Can you work these out from the model? Positions are in its coordinate system, mm. A direction names the side the tool comes from. Coordinates: 2 decimals unless noted, no trailing zeros. Order: outer loops, then holes, each group sorted by start corner. A loop starts at its lowest first (then second) coordinate and runs counter-clockwise, first axis right, second up. Notation, with made-up numbers: (64.25, 30.5) -> (90.25, 30.5) arc R33 ccw to (90.25, 62.5) -> close; hole circle Ø10 at (32.25, 33.5). An arc over 180 degrees is marked (long way). Write item = value, one per line. Start each with the question number.
Autodesk Inventor part; units mm, degrees
ref_plane "YZ Plane" through (0, 0, 0) normal (1, 0, 0) x (0, 1, 0)
ref_plane "XZ Plane" through (0, 0, 0) normal (0, 1, 0) x (-1, 0, 0)
ref_plane "XY Plane" through (0, 0, 0) normal (0, 0, 1) x (1, 0, 0)
sketch "Sketch1" plane through (0, 0, 0) normal (0, 1, 0) x (-1, 0, 0)
  circle A0 centre (25.2, -7) radius 1.35
  circle A1 centre (17.7, -7) radius 0.65
  circle A2 centre (15.2, -7) radius 0.65
  circle A3 centre (12.7, -7) radius 0.65
  line L0 (10, -7) -> (10, -8)
  line L1 (13, -11) -> (26, -11)
  line L2 (26, -3) -> (13, -3)
  line L3 (10, -6) -> (10, -7)
  arc A4 (13, -3) -> (10, -6) centre (13, -6) ccw
  arc A5 (10, -8) -> (13, -11) centre (13, -8) ccw
  line L4 (29, -14) -> (29, -18)
  line L5 (31, -20) -> (78, -20)
  line L6 (80, -18) -> (80, 4)
  line L7 (78, 6) -> (31, 6)
  line L8 (29, 4) -> (29, 0)
  arc A6 (26, -3) -> (29, 0) centre (26, 0) ccw
  arc A7 (29, -14) -> (26, -11) centre (26, -14) ccw
  arc A8 (31, 6) -> (29, 4) centre (31, 4) ccw
  arc A9 (80, 4) -> (78, 6) centre (78, 4) ccw
  arc A10 (78, -20) -> (80, -18) centre (78, -18) ccw
  arc A11 (29, -18) -> (31, -20) centre (31, -18) ccw
  point P0 (0, 0)
  point P1 (10, -3)
  point P2 (29, -7)
  point P3 (29, -20)
  point P4 (80, -20)
  point P5 (80, 6)
  point P6 (29, 6)
  dimension "d0" = 2.7
  dimension "d1" = 1.3
  dimension "d2" = 1.3
  dimension "d3" = 1.3
  dimension "d4" = 3
  dimension "d5" = 13
  dimension "d6" = 51
  dimension "d7" = 26
  dimension "d8" = 3
  dimension "d9" = 2
extrude "Extrusion1" add sketch "Sketch1" along normal blind 3
sketch "Sketch2" plane through (0, 3, 0) normal (0, 1, 0) x (1, 0, 0)
  line L0 (-77, 17) -> (-32, 17)
  line L1 (-32, 17) -> (-32, -3)
  line L2 (-32, -3) -> (-77, -3)
  line L3 (-77, -3) -> (-77, 17)
  line L4 (-78, 20) -> (-31, 20)
  line L5 (-29, 18) -> (-29, -4)
  line L6 (-41, -6) -> (-68, -6)
  line L7 (-80, -4) -> (-80, 18)
  arc A0 (-78, 20) -> (-80, 18) centre (-78, 18) ccw
  arc A1 (-29, 18) -> (-31, 20) centre (-31, 18) ccw
  arc A2 (-31, -6) -> (-29, -4) centre (-31, -4) ccw
  arc A3 (-80, -4) -> (-78, -6) centre (-78, -4) ccw
  line L8 (-77, -3) -> (-75.5, -3)
  line L9 (-75.5, -3) -> (-75.5, -1.5)
  circle A4 centre (-75.5, -1.5) radius 1
  line L10 (-32, 17) -> (-33.5, 17)
  line L11 (-33.5, 17) -> (-33.5, 15.5)
  circle A5 centre (-33.5, 15.5) radius 1
  line L12 (-49.42, 17) -> (-59.58, 17)
  line L13 (-59.58, 17) -> (-59.58, 14.46)
  line L14 (-59.58, 14.46) -> (-49.42, 14.46)
  line L15 (-49.42, 14.46) -> (-49.42, 17)
  line L16 (-78, -6) -> (-31, -6)
  line L17 (-77, -6) -> (-71, -6)
  line L18 (-71, -9) -> (-71, -9)
  line L19 (-74, -12) -> (-74, -12)
  line L20 (-77, -9) -> (-77, -6)
  line L21 (-32, -6) -> (-38, -6)
  line L22 (-38, -9) -> (-38, -9)
  line L23 (-35, -12) -> (-35, -12)
  line L24 (-32, -9) -> (-32, -6)
  arc A6 (-77, -9) -> (-74, -12) centre (-74, -9) ccw
  arc A7 (-74, -12) -> (-71, -9) centre (-74, -9) ccw
  arc A8 (-68, -6) -> (-71, -9) centre (-68, -9) ccw
  arc A9 (-38, -9) -> (-41, -6) centre (-41, -9) ccw
  arc A10 (-38, -9) -> (-35, -12) centre (-35, -9) ccw
  arc A11 (-35, -12) -> (-32, -9) centre (-35, -9) ccw
  circle A12 centre (-74, -9) radius 1.5
  circle A13 centre (-35, -9) radius 1.5
  line L25 (-77, -6) -> (-68, -6)
  line L26 (-41, -6) -> (-32, -6)
  point P0 (0, 0)
  point P1 (-38, -12)
  dimension "d12" = 45
  dimension "d13" = 20
  dimension "d14" = 2
  dimension "d15" = 1.5
  dimension "d16" = 1.5
  dimension "d17" = 2
  dimension "d18" = 1.5
  dimension "d19" = 1.5
  dimension "d20" = 2
  dimension "d22" = 10.16
  dimension "d23" = 2.54
  dimension "d24" = 3
  dimension "d25" = 3
  dimension "d26" = 3
extrude "Extrusion2" add sketch "Sketch2" against normal blind 3 contours L16 A8 A7 A6 L20 | L24 A11 A10 A9 L16
sketch "Sketch3" plane through (0, 3, 0) normal (0, 1, 0) x (1, 0, 0)
  line L0 (-77, 17) -> (-32, 17)
  line L1 (-32, 17) -> (-32, -3)
  line L2 (-32, -3) -> (-77, -3)
  line L3 (-77, -3) -> (-77, 17)
  line L4 (-78, 20) -> (-31, 20)
  line L5 (-29, 18) -> (-29, -4)
  line L6 (-41, -6) -> (-68, -6)
  line L7 (-80, -4) -> (-80, 18)
  arc A0 (-78, 20) -> (-80, 18) centre (-78, 18) ccw
  arc A1 (-29, 18) -> (-31, 20) centre (-31, 18) ccw
  arc A2 (-31, -6) -> (-29, -4) centre (-31, -4) ccw
  arc A3 (-80, -4) -> (-78, -6) centre (-78, -4) ccw
  line L8 (-77, -3) -> (-75.5, -3)
  line L9 (-75.5, -3) -> (-75.5, -1.5)
  circle A4 centre (-75.5, -1.5) radius 1
  line L10 (-32, 17) -> (-33.5, 17)
  line L11 (-33.5, 17) -> (-33.5, 15.5)
  circle A5 centre (-33.5, 15.5) radius 1
  line L12 (-49.42, 17) -> (-59.58, 17)
  line L13 (-59.58, 17) -> (-59.58, 14.46)
  line L14 (-59.58, 14.46) -> (-49.42, 14.46)
  line L15 (-49.42, 14.46) -> (-49.42, 17)
  line L16 (-78, -6) -> (-31, -6)
  line L17 (-77, -6) -> (-71, -6)
  line L18 (-71, -9) -> (-71, -9)
  line L19 (-74, -12) -> (-74, -12)
  line L20 (-77, -9) -> (-77, -6)
  line L21 (-32, -6) -> (-38, -6)
  line L22 (-38, -9) -> (-38, -9)
  line L23 (-35, -12) -> (-35, -12)
  line L24 (-32, -9) -> (-32, -6)
  arc A6 (-77, -9) -> (-74, -12) centre (-74, -9) ccw
  arc A7 (-74, -12) -> (-71, -9) centre (-74, -9) ccw
  arc A8 (-68, -6) -> (-71, -9) centre (-68, -9) ccw
  arc A9 (-38, -9) -> (-41, -6) centre (-41, -9) ccw
  arc A10 (-38, -9) -> (-35, -12) centre (-35, -9) ccw
  arc A11 (-35, -12) -> (-32, -9) centre (-35, -9) ccw
  circle A12 centre (-74, -9) radius 1.5
  circle A13 centre (-35, -9) radius 1.5
  line L25 (-77, -6) -> (-68, -6)
  line L26 (-41, -6) -> (-32, -6)
  point P0 (0, 0)
  point P1 (-38, -12)
  dimension "d29" = 45
  dimension "d30" = 20
  dimension "d31" = 2
  dimension "d32" = 1.5
  dimension "d33" = 1.5
  dimension "d34" = 2
  dimension "d35" = 1.5
  dimension "d36" = 1.5
  dimension "d37" = 2
  dimension "d38" = 10.16
  dimension "d39" = 2.54
  dimension "d40" = 3
  dimension "d41" = 3
  dimension "d42" = 3
extrude "Extrusion3" cut sketch "Sketch3" against normal blind 3 contours A4 | A5
(1) Imagine slicing it at B-B (y = 2.55). Count the separate pieces of the cut face and the enclosed holes in it, plus the area to 3 significant figures.
(2) Imagine slicing it at C-C (z = 1.5). Write out the boundary of the cut face in (x, y).
(3) If I drill on L1, parallel to X at y = 1.25, z = 9; L2, parallel to Z at x = -12.7, y = 1.7; L3, parallel to Z at x = -74, y = 1.55, over which ranges is the centre line in solid material (lowest first)? Write a range as from..to.
(4) Thinking about a two-plate mould opening in X: for faces 1 (the face through (-10.9, 1.48, -10.14)), 2 (the face through (-52, 0, -7)), 3 (the face through (-72.614, 1.521, 9.575)), which applies, +X half, -X half, draft (parallel to the pull), parting line (faces both ways), or undercut?
(5) Imagine slicing it at D-D (z = -7). Write out the boundary of the cut face in (x, y).
(6) Imagine slicing it at A-A (x = -25.2). Write out the boundary of the cut face in (y, z).
(7) For faces 4 (the face through (-18.32, 1.48, -7.2)), 5 (the face through (-19, 1, -11)), 6 (the face through (-79.43, 1.48, -19.4)), 7 (the face through (-77, 2, 8)), 8 (the face through (-55, 1, 6)), which set-ups out of +Z, -Z, +X, -X, +Y, -Y let a thin tool reach every point of the face, with its end or its side?
(8) For P1, Ø0.9, axis at y = 2, z = -15.5, coming from the +X side; P2, Ø1.5, axis at x = -55.5, y = 2, coming from the +Z side; P3, Ø1.5, axis at x = -19.5, y = 2, coming from the -Z side, each with a flat end and sliding along its axis, tell me the tip position at first contact or that it passes through.
Result set:
q1.separate_pieces = 1
q1.enclosed_holes = 8
q1.area = 1,510 mm2
q2.outline = (-80, 0) -> (-76.5, 0) -> (-76.5, 3) -> (-80, 3) -> close; (-74.5, 0) -> (-29, 0) -> (-29, 3) -> (-74.5, 3) -> close
q3.L1 = -77..-75.5, -72.5..-71, -38..-36.5, -33.5..-32
q3.L2 = -10.98..-7.65, -6.35..-3.02
q3.L3 = -20..7.5, 10.5..12
q4.face_1 = +X half
q4.face_2 = draft
q4.face_3 = undercut
q5.outline = (-80, 0) -> (-26.55, 0) -> (-26.55, 3) -> (-80, 3) -> close; (-23.85, 0) -> (-18.35, 0) -> (-18.35, 3) -> (-23.85, 3) -> close; (-17.05, 0) -> (-15.85, 0) -> (-15.85, 3) -> (-17.05, 3) -> close; (-14.55, 0) -> (-13.35, 0) -> (-13.35, 3) -> (-14.55, 3) -> close; (-12.05, 0) -> (-10, 0) -> (-10, 3) -> (-12.05, 3) -> close
q6.outline = (0, -11) -> (3, -11) -> (3, -8.35) -> (0, -8.35) -> close; (0, -5.65) -> (3, -5.65) -> (3, -3) -> (0, -3) -> close
q7.face_4 = +Y, -Y
q7.face_5 = -Z, +X, +Y, -Y
q7.face_6 = -Z, -X, +Y, -Y
q7.face_7 = +Z, -X, +Y, -Y
q7.face_8 = +Z, +Y, -Y
q8.P1 = -29
q8.P2 = 6
q8.P3 = -11
